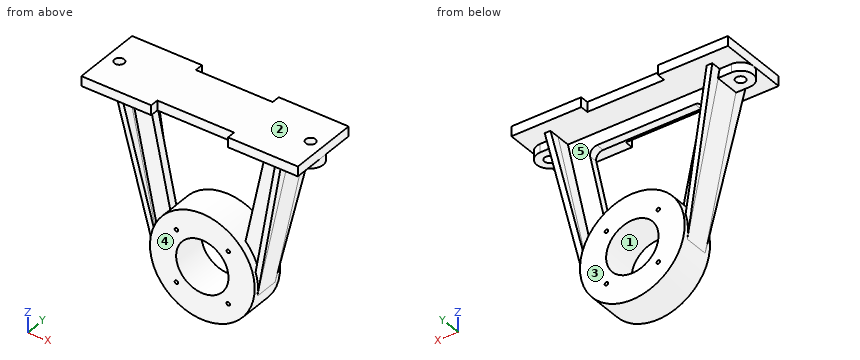
from build123d import *

# Parameters (mm, degrees)
BOSS_EXTRUDE1_DEPTH = 14
SKETCH2_R           = 75
SKETCH2_R_2         = 37.5
BOSS_EXTRUDE2_DEPTH = 25
SKETCH5_W           = 2.5
SKETCH5_H           = 50
CIRPATTERN1_COUNT   = 4
BOSS_EXTRUDE3_DEPTH = 17.5
BOSS_EXTRUDE4_DEPTH = 8
SKETCH9_R           = 7
BOSS_EXTRUDE5_DEPTH = 12
SKETCH10_R          = 7
CUT_EXTRUDE1_DEPTH  = 14
BOSS_EXTRUDE6_DEPTH = 12
FILLET1_R           = 10


with BuildPart() as part:
    # Sketch1 → Boss-Extrude1 (new body)
    with BuildSketch(Plane.XY):
        Polygon((-155, 50), (-55, 50), (-55, 38), (55, 38), (55, 50), (155, 50), (155, -50), (55, -50), (55, -38), (-55, -38), (-55, -50), (-155, -50), align=None)
    extrude(amount=BOSS_EXTRUDE1_DEPTH)



with BuildPart() as body_2:
    # Sketch2 → Boss-Extrude2 (new body, symmetric)
    with BuildSketch(Plane(origin=(0, 0, 0), x_dir=(1, 0, 0), z_dir=(0, 1, 0))):
        with Locations(Location((0, 206, 0), (0, 0, 270))):  # turned: the seam where the file's is
            Circle(SKETCH2_R)
        with Locations(Location((0, 206, 0), (0, 0, 270))):  # turned: the seam where the file's is
            Circle(SKETCH2_R_2, mode=Mode.SUBTRACT)
    extrude(amount=BOSS_EXTRUDE2_DEPTH, both=True)

    # Sketch5 → M6 Tapped Hole1 (revolve, cut)
    with BuildSketch(Plane(origin=(-37.123106012, 25, -243.123106012), x_dir=(0, 0, 1), z_dir=(1, 0, 0))):
        with Locations((1.25, 25)):
            Rectangle(SKETCH5_W, SKETCH5_H)
    m6_tapped_hole1 = revolve(axis=Axis((-37.123106012, 31.35, -243.123106012), (0, -1, 0)), mode=Mode.SUBTRACT)

    # CirPattern1: M6 Tapped Hole1 ×4 about axis
    cirpattern1_axis = Axis((0, 0, -206), (0, 1, 0))
    for i in range(1, CIRPATTERN1_COUNT):
        add(m6_tapped_hole1.rotate(cirpattern1_axis, i * 360 / CIRPATTERN1_COUNT), mode=Mode.SUBTRACT)


with BuildPart() as part_1:
    add(part.part)

    add(body_2.part)  # Boss-Extrude3 merges body 2
    # Sketch7 → Boss-Extrude3 (add, symmetric)
    with BuildSketch(Plane(origin=(0, 0, 0), x_dir=(1, 0, 0), z_dir=(0, 1, 0))):
        with BuildLine():
            Line((-111.824729359, 0), (-120, 0))
            Line((-120, 0), (-73.392065698, 221.446834387))
            ThreePointArc((-73.392065698, 221.446834387), (-74.975422623, 204.08010351), (-72.505303494, 186.81717004))
            Line((-72.505303494, 186.81717004), (-111.824729359, 0))
        make_face()
    boss_extrude3 = extrude(amount=BOSS_EXTRUDE3_DEPTH, both=True)

    # Sketch8 → Boss-Extrude4 (add)
    with BuildSketch(Plane(origin=(-114.909766558, 0, -24.185068462), x_dir=(-0.205957792, 0, 0.978560876), z_dir=(-0.978560876, 0, -0.205957792))):
        Polygon((-201.58354045, 17.5), (24.714935019, 32.5), (24.714935019, 17.5), align=None)
        Polygon((24.714935019, -32.5), (24.714935019, -17.5), (-201.58354045, -17.5), align=None)
    boss_extrude4 = extrude(amount=-BOSS_EXTRUDE4_DEPTH)

    # Sketch9 → Boss-Extrude5 (add)
    with BuildSketch(Plane(origin=(0, 0, 0), x_dir=(-1, 0, 0), z_dir=(0, 0, -1))):
        with BuildLine():
            Line((111.824729359, 18), (111.824729359, -18))
            Line((111.824729359, -18), (137, -18))
            ThreePointArc((137, -18), (155, 0), (137, 18))
            Line((137, 18), (111.824729359, 18))
        make_face()
        with Locations((137, 0)):
            Circle(SKETCH9_R, mode=Mode.SUBTRACT)
    boss_extrude5 = extrude(amount=BOSS_EXTRUDE5_DEPTH)

    # Sketch10 → Cut-Extrude1 (cut)
    with BuildSketch(Plane(origin=(0, 0, 0), x_dir=(-1, 0, 0), z_dir=(0, 0, -1))):
        with Locations((137, 0)):
            Circle(SKETCH10_R)
    cut_extrude1 = extrude(amount=-CUT_EXTRUDE1_DEPTH, mode=Mode.SUBTRACT)

    # Mirror3: Boss-Extrude3, Boss-Extrude4, Boss-Extrude5, Cut-Extrude1 across plane
    add(boss_extrude3.mirror(Plane(origin=(0, 0, 0), x_dir=(0, 0, 1), z_dir=(1, 0, 0))))
    add(boss_extrude4.mirror(Plane(origin=(0, 0, 0), x_dir=(0, 0, 1), z_dir=(1, 0, 0))))
    add(boss_extrude5.mirror(Plane(origin=(0, 0, 0), x_dir=(0, 0, 1), z_dir=(1, 0, 0))))
    add(cut_extrude1.mirror(Plane(origin=(0, 0, 0), x_dir=(0, 0, 1), z_dir=(1, 0, 0))), mode=Mode.SUBTRACT)

    # Sketch13 → Boss-Extrude6 (add)
    with BuildSketch(Plane(origin=(0, -2, 0), x_dir=(1, 0, 0), z_dir=(0, 1, 0))):
        with BuildLine():
            Line((-111.824729359, 0), (-72.505303494, 186.81717004))
            ThreePointArc((-72.505303494, 186.81717004), (-65.31598907, 169.137802944), (-53.897144884, 153.845443407))
            Line((-53.897144884, 153.845443407), (-82.488547055, 18))
            Line((-82.488547055, 18), (82.488547055, 18))
            Line((82.488547055, 18), (53.897144884, 153.845443407))
            ThreePointArc((53.897144884, 153.845443407), (65.31598907, 169.137802944), (72.505303494, 186.81717004))
            Line((72.505303494, 186.81717004), (111.824729359, 0))
            Line((111.824729359, 0), (55, 0))
            Line((55, 0), (-111.824729359, 0))
        make_face()
    extrude(amount=-BOSS_EXTRUDE6_DEPTH)

    # Fillet1
    fillet1_edges = [part_1.edges().sort_by_distance(p)[0] for p in [
        (-82.488547055, -8, -18),
        (82.488547055, -8, -18),
    ]]
    fillet(fillet1_edges, radius=FILLET1_R)


solid = part_1.part
The listing builds one solid part. Answer for the finished solid, in the listing's coordinates (mm). Face numbers are marked on the shaded views. A direction names the side the tool comes from. Give positions to 0.01 mm unless a question says otherwise; leave off trailing zeros. Loops run counter-clockwise (first coordinate to the right, second up) from the corner with the lowest first, then second, coordinate; pieces in that order, holes last. Notation, with made-up numbers: M 34.5,-27.75 L 80.5,-27.75 A28 ccw 80.5,8.25 Z; hole C 16,-2.75 d4. An arc over 180 degrees is marked long. Answer as CSV lines item,"result".
Item 1: The part is cut by section C-C (z = -229). Give the vertices of the cut face in (x, y).
Values follow:
outline,"M -71.39,-25 L -29.62,-25 L -29.62,25 L -71.39,25 Z; M 29.62,-25 L 71.39,-25 L 71.39,25 L 29.62,25 Z"
Item 2: The part is cut by section D-D (x = 93). Give the vertices of the cut face in (y, z), and give its area (3 significant figures).
Values follow:
outline,"M -50,0 L -14,0 L -14,-89.44 L -26.33,-89.44 L -23.81,-128.28 L 23.81,-128.28 L 26.33,-89.44 L -2,-89.44 L -2,0 L 50,0 L 50,14 L -50,14 Z"
area,"4,420 mm^2"
Item 3: Which of the six approach directions +Z, -Z, +X, -X, +Y, -Y give full straight-line access (tool end or side, diameter ignored) to the marked faces 3, 4 and 5?
Values follow:
face 3,"-Z, +X, -X, +Y"
face 4,"-Z, +X, -X, -Y"
face 5,"+Y"
Item 4: Straight lines are drawn through the part: line 1 along Z through (x, y) = (38, -16); line 2 along Y through (x, z) = (137, -7); line 3 along Z through (x, y) = (13, -1.5). For each, find the intervals that lie inside material, in ascending order. Write a range as [from, to].
Values follow:
line 1,"z = [-270.66, -245.46], [-240.78, -171.22], [-166.54, -141.34], [0, 14]"
line 2,"y = [-18, -7], [7, 18]"
line 3,"z = [-279.86, -241.17], [-170.83, -132.14], [0, 14]"
Item 5: Given pin 1 Ø8 at (x, z) = (90.5, -118.5) entering from +Y; pin 2 Ø11 at (x, y) = (128.5, -6.5) entering from -Z; pin 3 Ø4 at (x, y) = (-48.5, 3) entering from -Z, each flat-ended and moving along its own axis, determine where each tip first touches the part or whether it passes through.
Values follow:
pin 1,"stops at y = 24.68"
pin 2,"stops at z = -12"
pin 3,"stops at z = -264.85"
Item 6: The part is cut by section B-B (x = 17). Give the vertices of the cut face in (y, z).
Values follow:
outline,"M -38,0 L -14,0 L -14,-18 L -2,-18 L -2,0 L 38,0 L 38,14 L -38,14 Z; M -25,-279.05 L 25,-279.05 L 25,-239.43 L -25,-239.43 Z; M -25,-172.57 L 25,-172.57 L 25,-132.95 L -25,-132.95 Z"
Item 7: The mould has two halves that part along X. Classify the marked faces 1 and 2: released by +X, released by -X, zero draft, split by the parting line, or undercut.
Values follow:
face 1,"undercut"
face 2,"zero draft"
Item 8: The part is cut by section A-A (z = -83). Give the vertices of the cut face in (x, y), and give its area (3 significant figures).
Values follow:
outline,"M -102.53,-26.88 L -94.36,-26.77 L -94.36,-14 L -68.81,-14 L -68.81,-2 L -94.36,-2 L -94.36,26.77 L -102.53,26.88 Z; M 68.81,-14 L 94.36,-14 L 94.36,-26.77 L 102.53,-26.88 L 102.53,26.88 L 94.36,26.77 L 94.36,-2 L 68.81,-2 Z"
area,"1,490 mm^2"
